from build123d import *

# Parameters (mm, degrees)
SKETCH1_W                 = 25.41
SKETCH1_H                 = 12
BOSS_EXTRUDE1_DEPTH       = 6
SKETCH2_R                 = 2.42
CUT_EXTRUDE1_DEPTH        = 25.41
SKETCH4_W                 = 4.522418919
SKETCH4_H                 = 1.5
CUT_EXTRUDE2_DEPTH        = 25.41
F_2_56_TAPPED_HOLE1_D     = 2.000000064
F_2_56_TAPPED_HOLE1_DEPTH = 2.649139362
F_2_56_TAPPED_HOLE1_TIP   = 0.600860638
F_0_80_TAPPED_HOLE1_D     = 1.19126
F_0_80_TAPPED_HOLE1_DEPTH = 3.642109389
F_0_80_TAPPED_HOLE1_TIP   = 0.357890611


with BuildPart() as part:
    # Sketch1 → Boss-Extrude1 (new body)
    with BuildSketch(Plane(origin=(0, 0, 0), x_dir=(1, 0, 0), z_dir=(0, 1, 0))):
        with Locations((12.705, 6)):
            Rectangle(SKETCH1_W, SKETCH1_H)
    extrude(amount=BOSS_EXTRUDE1_DEPTH)

    # Sketch2 → Cut-Extrude1 (cut)
    with BuildSketch(Plane.ZY):
        with Locations((-6, 6)):
            Circle(SKETCH2_R)
    extrude(amount=-CUT_EXTRUDE1_DEPTH, mode=Mode.SUBTRACT)

    # Sketch4 → Cut-Extrude2 (cut)
    with BuildSketch(Plane.ZY):
        with Locations((-9.738790541, 5.25)):
            Rectangle(SKETCH4_W, SKETCH4_H)
    extrude(amount=-CUT_EXTRUDE2_DEPTH, mode=Mode.SUBTRACT)

    # #2-56 Tapped Hole1
    with Locations(Plane(origin=(0, 0, 0), x_dir=(-1, 0, 0), z_dir=(0, -1, 0))):
        with Locations((-23.91, 6), (-1.5, 6)):
            Hole(F_2_56_TAPPED_HOLE1_D / 2, depth=F_2_56_TAPPED_HOLE1_DEPTH)
            with Locations((0, 0, -(F_2_56_TAPPED_HOLE1_DEPTH + F_2_56_TAPPED_HOLE1_TIP / 2))):  # 118° drill point
                Cone(0, F_2_56_TAPPED_HOLE1_D / 2, F_2_56_TAPPED_HOLE1_TIP, mode=Mode.SUBTRACT)

    # #0-80 Tapped Hole1
    with Locations(Plane(origin=(0, 6, 0), x_dir=(1, 0, 0), z_dir=(0, 1, 0))):
        with Locations((5.082, 1.79), (10.164, 1.79), (15.246, 1.79), (20.328, 1.79)):
            Hole(F_0_80_TAPPED_HOLE1_D / 2, depth=F_0_80_TAPPED_HOLE1_DEPTH)
            with Locations((0, 0, -(F_0_80_TAPPED_HOLE1_DEPTH + F_0_80_TAPPED_HOLE1_TIP / 2))):  # 118° drill point
                Cone(0, F_0_80_TAPPED_HOLE1_D / 2, F_0_80_TAPPED_HOLE1_TIP, mode=Mode.SUBTRACT)


solid = part.part
Could you check a few things on this model? Use its own coordinates, in mm. A direction names the side the tool comes from. Coordinates: 2 decimals unless noted, no trailing zeros. Order: outer loops, then holes, each group sorted by start corner. A loop starts at its lowest first (then second) coordinate and runs counter-clockwise, first axis right, second up. Notation, with made-up numbers: (7, 29) -> (40, 29) arc R29 cw to (40, 53) -> close; hole circle Ø4 at (87.25, 81.5). An arc over 180 degrees is marked (long way). One line per item, written item: value. Start each with the question number.
1) I'm going to push flat-ended pins straight in: pin 1 (4.5 mm diameter, centred on x = 12.5, z = -10, fed in from +Y); pin 2 (1.1 mm diameter, centred on x = 20.328, z = -1.79, fed in from +Y). Where does each tip first touch, or does it pass through?
2) We'd pull the mould along Z, two halves only. Please class faces 1 (the flat face through (13, 4.5, -10)), 2 (the flat face through (13, 2, -12)), 3 (the conical face through (23.75, 3.146, -5.933)): +Z half, -Z half, draft (parallel to the pull), parting line (faces both ways), or undercut.
3) Imagine slicing it at A-A on y = 1.35. List the corners of the cut face in (x, z) for me, plus the area to 3 significant figures.
4) Imagine slicing it at B-B on x = 19.5. List the corners of the cut face in (y, z) for me.
5) Which directions (+Z, -Z, +X, -X, +Y, -Y) give clear straight access to the entire face, cutting with the end or side of a thin tool? Please do faces 4 (the flat face through (13, 0, -6)), 5 (the cylindrical face through (22.91, 1.34, -6.04)), 6 (the cylindrical face through (10.64, 4.15, -1.43)).
6) If I drill on L1, parallel to X at y = 0.7, z = -6; L2, parallel to Z at x = 23.91, y = 2.1; L3, parallel to X at y = 1.65, z = -5.25, over which ranges is the centre line in solid material (lowest first)? Write a range as [from, to].
7) Imagine slicing it at C-C on z = -9.5. List the corners of the cut face in (x, y) for me, plus the area to 3 significant figures.
8) Imagine slicing it at D-D on y = 4.85. List the corners of the cut face in (x, z) for me.
Answer list:
1. pin 1: stops at y = 4.5
1. pin 2: stops at y = 2.33
2. face 1: draft
2. face 2: -Z half
2. face 3: undercut
3. outline: (0, -12) -> (25.41, -12) -> (25.41, 0) -> (0, 0) -> close; hole circle Ø2 at (1.5, -6); hole circle Ø2 at (23.91, -6)
3. area: 299 mm2
4. outline: (0, -12) -> (4.5, -12) -> (4.5, -7.9) arc R2.42 cw to (6, -3.58) -> (6, 0) -> (0, 0) -> close
5. face 4: +Z, -Z, +X, -X, -Y
5. face 5: -Y
5. face 6: +Y
6. L1: x = [0, 0.5], [2.5, 22.91], [24.91, 25.41]
6. L2: z = [-12, -7], [-5, 0]
6. L3: x = [0, 0.84], [2.16, 23.25], [24.57, 25.41]
7. outline: (0, 0) -> (25.41, 0) -> (25.41, 4.5) -> (0, 4.5) -> close
7. area: 114 mm2
8. outline: (0, -3.87) -> (25.41, -3.87) -> (25.41, 0) -> (0, 0) -> close; hole circle Ø1.19 at (5.08, -1.79); hole circle Ø1.19 at (10.16, -1.79); hole circle Ø1.19 at (15.25, -1.79); hole circle Ø1.19 at (20.33, -1.79)
